CAD build for the part. Positions are in the model's coordinates, mm. A direction names the side the tool comes from. Coordinates: 2 decimals unless noted, no trailing zeros. Order: outer loops, then holes, each group sorted by start corner. A loop starts at its lowest first (then second) coordinate and runs counter-clockwise, first axis right, second up. Notation, with made-up numbers: (-28.5, 11) - (16.5, 11) arc R18 cw to (16.5, 40) - close; hole circle Ø6 at (71, 6). An arc over 180 degrees is marked (long way). Write each question's results on one line, items separated by ' | '. Start each with the question number.
Q1. Band-saw the part on A-A, the plane y = -22. Write the cut outline in (x, z), then the cut area to 3 significant figures.
Q2. Wall check: probe 1 along X at (y, z) = (29, 70); probe 2 along Z at (x, y) = (33, -10). Give the ranges that are in metal, low to high.
Q3. Pin check, flat tips, straight feed: P1, Ø5, axis at x = -34.5, y = -9, coming from the -Z side; P2, Ø8, axis at x = -1, y = 27.5, coming from the +Z side. Stop position of each tip, or through.
Q4. Pull direction Z, two halves, no side cores. Call faces 4 (the flat face through (-35, -31.75, 38)), 5 (the flat face through (0, -35, 6.35)), 6 (the flat face through (0, 31.75, 3)), 7 (the flat face through (-34, 1, 0)): released by +Z, released by -Z, zero draft, split by the parting line, or undercut.
Q5. Which spindle directions (+Z, -Z, +X, -X, +Y, -Y) get a long thin tool onto all of the face, cutting with end or side? Do faces 1 (the flat face through (-31.75, 0, 3)), 2 (the flat face through (35, 0, 69.85)), 3 (the flat face through (-31.75, 35, 38)). Say none if no direction does.
```python
from build123d import *

# Parameters (mm, degrees)
F0_W     = 76.2
F0_H     = 76.2
F1_DEPTH = 76.2
F2_W     = 63.5
F2_H     = 63.5
F3_DEPTH = 76.2
F4_W     = 63.5
F4_H     = 63.5
F5_DEPTH = 76.2
F6_W     = 63.5
F6_H     = 63.5
F7_DEPTH = 76.2


with BuildPart() as f1:
    # F0 (on Top) → F1 (new body)
    with BuildSketch(Plane.XY):
        Rectangle(F0_W, F0_H)
    extrude(amount=F1_DEPTH)

    # F2 (on face) → F3 (cut)
    with BuildSketch(Plane.XZ.offset(38.1)):
        with Locations((0, 38.1)):
            Rectangle(F2_W, F2_H)
    extrude(amount=-F3_DEPTH, mode=Mode.SUBTRACT)

    # F4 (on face) → F5 (cut)
    with BuildSketch(Plane(origin=(-38.1, 0, 0), x_dir=(0, -1, 0), z_dir=(-1, 0, 0))):
        with Locations((0, 38.1)):
            Rectangle(F4_W, F4_H)
    extrude(amount=-F5_DEPTH, mode=Mode.SUBTRACT)

    # F6 (on face) → F7 (cut)
    with BuildSketch(Plane(origin=(0, 0, 0), x_dir=(1, 0, 0), z_dir=(0, 0, -1))):
        Rectangle(F6_W, F6_H)
    extrude(amount=-F7_DEPTH, mode=Mode.SUBTRACT)


solid = f1.part
```
Results below:
1) outline: (-38.1, 0) - (-31.75, 0) - (-31.75, 6.35) - (-38.1, 6.35) - close; (-38.1, 69.85) - (-31.75, 69.85) - (-31.75, 76.2) - (-38.1, 76.2) - close; (31.75, 0) - (38.1, 0) - (38.1, 6.35) - (31.75, 6.35) - close; (31.75, 69.85) - (38.1, 69.85) - (38.1, 76.2) - (31.75, 76.2) - close | area: 161 mm²
2) probe 1: x = -38.1 to -31.75, 31.75 to 38.1 | probe 2: z = 0 to 6.35, 69.85 to 76.2
3) P1: stops at z = 0 | P2: passes through
4) face 4: undercut | face 5: undercut | face 6: zero draft | face 7: released by -Z
5) face 1: +Z, -Z | face 2: +X, -X | face 3: +Y, -Y
